Input: part model. Units: mm. Frame: model coordinates. A direction names the side the tool comes from. Round coordinates to 2 decimals unless told otherwise and drop trailing zeros. Loops run counter-clockwise (first coordinate to the right, second up) from the corner with the lowest first, then second, coordinate; pieces in that order, holes last. Notation, with made-up numbers: (24, -36.5) -> (46, -36.5) arc R20 cw to (46, -9.5) -> close; hole circle Ø10 at (57, 76). An arc over 180 degrees is marked (long way). Answer in a Markdown table with one row per item. Add a question column.
Q1. Ray query, L1, parallel to X at y = 236, z = 0 (3 decimals); L2, parallel to Y at x = -17.5, z = -52.5; L3, parallel to X at y = 229, z = 0. Return the intervals inside material, ascending. Write a range as from..to.
Q2. Mould query, pull axis X, two halves, no side actions, for faces 5 (the face through (50.623, 235.036, -26.33)), 6 (the face through (32, 0, 10)), 7 (the face through (17.48, 9.503, 22.797)). Classes: pulls with the +X half, pulls with the -X half, needs draft (parallel to the pull), parting line crosses it, or undercut.
Q3. Pin query (flat end, axial travel): pin 1 (3 mm diameter, centred on x = -35, z = -26, fed in from +Y); pin 2 (6 mm diameter, centred on x = 6, y = 203.5, fed in from -Z); pin 3 (4 mm diameter, centred on x = 9, z = -41, fed in from +Y). Return the tip coordinate at first contact, or that it passes through.
Q4. Section A-A, the plane y = 172. Output: boundary loops of the cut face in (x, z) (3 decimals).
Q5. Reachability of faces 1 (the face through (-1.29, 5.52, 29.34)), 2 (the face through (-36.48, 235.96, 39.78)), 3 (the face through (4, 210.947, -51)), 4 (the face through (23.129, 23.052, -55.784)) from +Z, -Z, +X, -X, +Y, -Y: full face, straight path, thin tool, end or side. Return the list, or none.
```python
from build123d import *

# Parameters (mm, degrees)
FILLET1_R = 3.175
FILLET5_R = 12.7
FILLET6_R = 3.175


with BuildPart() as part:
    # Sketch1 → Revolve1 (revolve)
    with BuildSketch(Plane.XY, mode=Mode.PRIVATE) as revolve1_sk:
        Polygon((28.7274, 7.9375), (29.36875, 7.9375), (29.36875, 0), (60.3885, 0), (60.3885, 7.6835), (58.8645, 7.6835), (58.8645, 20.6375), (60.3885, 20.6375), (60.3885, 25.4), (57.0611, 25.4), (57.0611, 197.612), (57.0611, 203.962), (50.8635, 203.962), (50.8635, 210.947), (57.0611, 210.947), (57.0611, 226.822), (54.8386, 226.822), (54.8386, 233.426), (57.0611, 233.426), (57.0611, 236.601), (53.975, 236.601), (53.975, 235.331), (50, 235.331), (50, 224.25700005), (51.75, 224.25700005), (51.75, 221.107), (50, 221.107), (50, 217.297), (47.625, 213.183379332), (47.625, 30.1625), (28.7274, 26.9875), (28.7274, 26.289), (30.9499, 26.289), (30.9499, 19.685), (28.7274, 19.685), (28.7274, 18.0975), (34.925, 18.0975), (34.925, 11.1125), (28.7274, 11.1125), align=None)
    revolve(revolve1_sk.sketch.rotate(Axis((0, 0, 0), (0, 1, 0)), 90), axis=Axis((0, 0, 0), (0, 1, 0)))

    # Fillet1
    fillet1_edges = [part.edges().sort_by_distance(p)[0] for p in [
        (0, 30.1625, 47.625),
    ]]
    fillet(fillet1_edges, radius=FILLET1_R)

    # Fillet5
    # the kernel refuses this fillet: 12.7 mm, written as the material it takes off along each edge
    with BuildSketch(Plane(origin=(0, 0, 0), x_dir=(0, 0, -1), z_dir=(1, 0, 0))) as fillet5_piece_1:
        with BuildLine():
            CenterArc((48.721249778, 12.7), FILLET5_R, 270, 66.734025938)
            Line((60.3885, 7.6835), (60.621845004, 7.58317))
            ThreePointArc((60.621845004, 7.58317), (60.6425, 3.84175), (60.6425, 0))
            Line((60.6425, 0), (60.3885, -0.254))
            Line((60.3885, -0.254), (48.721249778, -0.254))
            Line((48.721249778, -0.254), (48.721249778, 0))
        make_face()
    revolve(axis=Axis((0, 0, 0), (0, 1, 0)), mode=Mode.SUBTRACT)

    # Fillet6
    fillet6_edges = [part.edges().sort_by_distance(p)[0] for p in [
        (0, 0, 29.36875),
    ]]
    fillet(fillet6_edges, radius=FILLET6_R)


solid = part.part
```
Answer block:
| question | item | result |
|---|---|---|
| 1 | L1 | -57.061..-53.975, 53.975..57.061 |
| 1 | L2 | 1.86..203.96, 210.95..226.82, 233.43..236.6 |
| 1 | L3 | -54.84..-50, 50..54.84 |
| 2 | face 5 | parting line crosses it |
| 2 | face 6 | needs draft |
| 2 | face 7 | undercut |
| 3 | pin 1 | y = 29.74 |
| 3 | pin 2 | z = -56.98 |
| 3 | pin 3 | y = 29.55 |
| 4 | outline | circle Ø114.122 at (0, 0); hole circle Ø95.25 at (0, 0) |
| 5 | face 1 | -Y |
| 5 | face 2 | +Y |
| 5 | face 3 | none |
| 5 | face 4 | +Y, -Y |
